Check sheet for the drawn part. Datum: minimum x, y, z corner. Units: mm. A direction names the side the tool comes from. Coordinates: 2 decimals unless noted, no trailing zeros. Order: outer loops, then holes, each group sorted by start corner. A loop starts at its lowest first (then second) coordinate and runs counter-clockwise, first axis right, second up. Notation, with made-up numbers: (64.5, 17.5) - (75.5, 17.5) arc R25 ccw to (75.5, 43.5) - close; hole circle Ø1 at (15.25, -32). An arc over 180 degrees is marked (long way). Return JSON: item names as keys, results as strings. Group by question number.
Item 1: Section check A-A on z = 25.4. Enter the section's corners in (x, y), then the cut area to 3 significant figures.
Item 2: Draft check along Y on the marked faces 1, 2 and 3. Enter one of: pulls with the +Y half, pulls with the -Y half, needs draft (parallel to the pull), parting line crosses it, or undercut.
Item 3: Scan lines: probe 1 along X at (y, z) = (17.5, 19); probe 2 along Y at (x, z) = (41.5, 24.5) (1 decimal); probe 3 along Z at (x, y) = (49.5, 18) (1 decimal). Record each from-to range of solid material in increasing order.
Item 4: Section check C-C on z = 4. Enter the section's corners in (x, y), then the cut area to 3 significant figures.
Item 5: Tool access check on the marked faces 4, 5, 6 and 7. Record the directions out of +Z, -Z, +X, -X, +Y, -Y that give a thin tool (end or side, any length) a straight path to the whole face; none if there is none.
Item 6: Section check D-D on y = 13.5. Enter the section's corners in (x, z) (1 decimal).
Item 7: Gauge pin test, flat ends, axial feed: pin 1 (3 mm diameter, centred on y = 10, z = 18, fed in from +X); pin 2 (5 mm diameter, centred on x = 31, y = 8, fed in from -Z); pin 3 (10 mm diameter, centred on y = 26, z = 20, fed in from -X); pin 4 (1.5 mm diameter, centred on x = 27.5, z = 15, fed in from -Y). Record the tip position at first contact, or that the pin passes through.
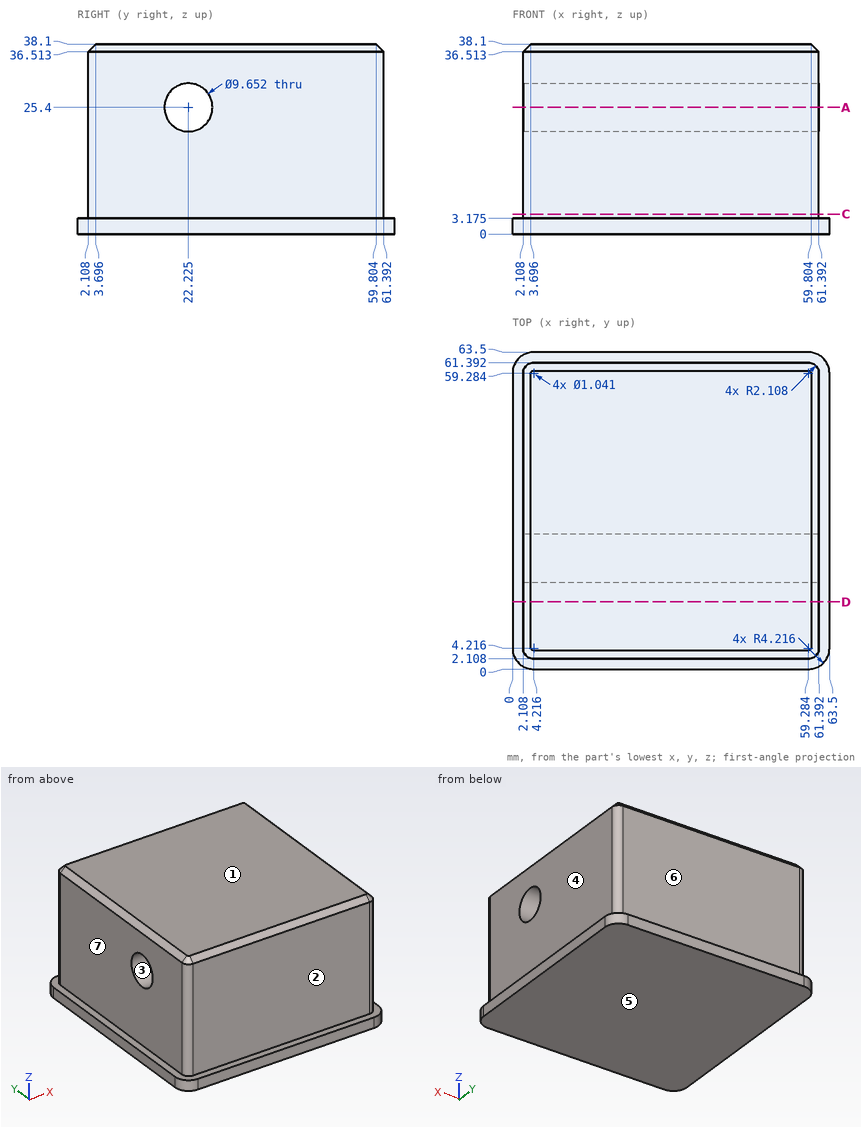
Computed:
{
 "1": {"outline": "(2.11, 4.22) arc R2.11 ccw to (4.22, 2.11) - (59.28, 2.11) arc R2.11 ccw to (61.39, 4.22) - (61.39, 17.4) - (2.11, 17.4) - close; (2.11, 27.05) - (61.39, 27.05) - (61.39, 59.28) arc R2.11 ccw to (59.28, 61.39) - (4.22, 61.39) arc R2.11 ccw to (2.11, 59.28) - close", "area": "2,940 mm²"},
 "2": {"face 1": "needs draft", "face 2": "pulls with the -Y half", "face 3": "undercut"},
 "3": {"probe 1": "x = 2.11 to 61.39", "probe 2": "y = 2.1 to 17.5, 27 to 61.4", "probe 3": "z = 0 to 23.1, 27.7 to 38.1"},
 "4": {"outline": "(2.11, 4.22) arc R2.11 ccw to (4.22, 2.11) - (59.28, 2.11) arc R2.11 ccw to (61.39, 4.22) - (61.39, 59.28) arc R2.11 ccw to (59.28, 61.39) - (4.22, 61.39) arc R2.11 ccw to (2.11, 59.28) - close", "area": "3,510 mm²"},
 "5": {"face 4": "+Z, +X, +Y, -Y", "face 5": "-Z, +X, -X, +Y, -Y", "face 6": "+Z, +X, -X, +Y", "face 7": "+Z, -X, +Y, -Y"},
 "6": {"outline": "(0, 0) - (63.5, 0) - (63.5, 3.2) - (61.4, 3.2) - (61.4, 36.5) - (59.8, 38.1) - (3.7, 38.1) - (2.1, 36.5) - (2.1, 3.2) - (0, 3.2) - close"},
 "7": {"pin 1": "stops at x = 61.39", "pin 2": "stops at z = 0", "pin 3": "stops at x = 2.11", "pin 4": "stops at y = 2.11"}
}
